Read the model definition and answer for the solid it produces. Units are mm, in the model's axes. Face numbers are marked on the shaded views. A direction names the side the tool comes from. Coordinates: 2 decimals unless noted, no trailing zeros. Write item = value, one per line.
from build123d import *

# Parameters (mm, degrees)
BOSS_EXTRUDE1_DEPTH  = 17.5
CUT_EXTRUDE1_DEPTH   = 15.5
CUT_EXTRUDE3_REACH   = 38.949
SKETCH4_R            = 8
SKETCH4_4_R          = 1
SKETCH4_4_W          = 20
SKETCH4_4_H          = 5
BOSS_EXTRUDE2_DEPTH  = 7
FILLET1_R            = 1
FILLET2_R            = 1.5
BOSS_EXTRUDE3_DEPTH  = 2
SKETCH6_W            = 11
SKETCH6_H            = 2
BOSS_EXTRUDE4_DEPTH  = 0.75
SKETCH11_R           = 8
BOSS_EXTRUDE11_DEPTH = 0.5
SKETCH14_W           = 11
SKETCH14_H           = 11
BOSS_EXTRUDE12_DEPTH = 2
BOSS_EXTRUDE13_DEPTH = 1
SKETCH6_4_W          = 11
SKETCH6_4_H          = 2.5
CUT_EXTRUDE6_DEPTH   = 0.3
SKETCH16_W           = 11
SKETCH16_H           = 2
BOSS_EXTRUDE14_DEPTH = 0.75
SKETCH16_3_W         = 11
SKETCH16_3_H         = 2.5
CUT_EXTRUDE7_DEPTH   = 0.3
CUT_EXTRUDE8_REACH   = 59.044
FILLET3_R            = 1
CHAMFER1_SIZE        = 0.5
CHAMFER3_SIZE        = 1


with BuildPart() as part:
    # Sketch1 → Boss-Extrude1 (new body)
    with BuildSketch(Plane(origin=(0, 0, 0), x_dir=(1, 0, 0), z_dir=(0, 1, 0))):
        Polygon((-15, 20), (15, 20), (15, -20), (15, -30), (-15, -30), (-15, -20), align=None)
    extrude(amount=BOSS_EXTRUDE1_DEPTH)

    # Sketch2 → Cut-Extrude1 (cut)
    with BuildSketch(Plane(origin=(0, 17.5, 0), x_dir=(1, 0, 0), z_dir=(0, 1, 0))):
        Polygon((-13, 18), (13, 18), (13, -18), (13, -28), (-13, -28), (-13, -18), align=None)
    extrude(amount=-CUT_EXTRUDE1_DEPTH, mode=Mode.SUBTRACT)

    # Sketch4 → Cut-Extrude3 (cut, up to next)
    with BuildSketch(Plane(origin=(0, 2, 0), x_dir=(1, 0, 0), z_dir=(0, 1, 0)), mode=Mode.PRIVATE) as cut_extrude3_sk1:
        with Locations(Location((0, 3.5, 0), (0, 0, 270))):
            Circle(SKETCH4_R)
    cut_extrude3_tool1 = extrude(cut_extrude3_sk1.sketch, amount=-CUT_EXTRUDE3_REACH, mode=Mode.PRIVATE) & part.part
    add(cut_extrude3_tool1.solids().sort_by_distance((0, 2, -3.5))[0], mode=Mode.SUBTRACT)

    # Sketch4<4> → Boss-Extrude2 (add)
    # profile 1 of 2: a face of its own
    with BuildSketch(Plane(origin=(0, 2, 0), x_dir=(1, 0, 0), z_dir=(0, 1, 0))):
        Polygon((10, 16), (-10, 16), (-10, 11), (-5.998750655, 11), (-3.877430311, 13.121320344), (3.877430311, 13.121320344), (5.998750655, 11), (10, 11), align=None)
        with Locations(Location((-7.5, 13.5, 0), (0, 0, 270))):
            Circle(SKETCH4_4_R, mode=Mode.SUBTRACT)
        with Locations(Location((7.5, 13.5, 0), (0, 0, 270))):
            Circle(SKETCH4_4_R, mode=Mode.SUBTRACT)
    # profile 2 of 2: a face of its own
    with BuildSketch(Plane(origin=(0, 2, 0), x_dir=(1, 0, 0), z_dir=(0, 1, 0))):
        with Locations((0, -13.5)):
            Rectangle(SKETCH4_4_W, SKETCH4_4_H)
        with Locations(Location((7.5, -13.5, 0), (0, 0, 270))):
            Circle(SKETCH4_4_R, mode=Mode.SUBTRACT)
        with Locations(Location((-7.5, -13.5, 0), (0, 0, 270))):
            Circle(SKETCH4_4_R, mode=Mode.SUBTRACT)
    extrude(amount=BOSS_EXTRUDE2_DEPTH)

    # Fillet1
    fillet1_edges = [part.edges().sort_by_distance(p)[0] for p in [
        (-4.938090483, 2, -12.060660172),
        (0, 2, -13.121320344),
        (-10, 2, -13.5),
        (-7.999375327, 2, -11),
        (0, 2, -16),
        (10, 2, -13.5),
        (7.999375327, 2, -11),
        (4.938090483, 2, -12.060660172),
        (-10, 2, 13.5),
        (0, 2, 16),
        (0, 2, 11),
        (10, 2, 13.5),
    ]]
    fillet(fillet1_edges, radius=FILLET1_R)

    # Fillet2
    fillet2_edges = [part.edges().sort_by_distance(p)[0] for p in [
        (15, 8.75, 30),
        (-15, 8.75, 30),
        (-15, 8.75, -20),
        (15, 8.75, -20),
        (0, 0, 30),
        (-15, 0, 5),
        (0, 0, -20),
        (15, 0, 5),
    ]]
    fillet(fillet2_edges, radius=FILLET2_R)

    # Sketch5 → Boss-Extrude3 (add)
    with BuildSketch(Plane(origin=(-13, 0, 0), x_dir=(0, 0, -1), z_dir=(1, 0, 0))):
        Polygon((-12, 17.5), (-18, 17.5), (-23, 17.5), (-23, 12), (-12, 12), align=None)
        Polygon((-23, 17.5), (-18, 17.5), (-12, 17.5), (-12, 23), (-23, 23), align=None)
    extrude(amount=BOSS_EXTRUDE3_DEPTH)

    # Sketch6 → Boss-Extrude4 (add)
    with BuildSketch(Plane.ZY.offset(13)):
        with Locations((17.5, 22)):
            Rectangle(SKETCH6_W, SKETCH6_H)
    extrude(amount=BOSS_EXTRUDE4_DEPTH)

    # Sketch11 → Boss-Extrude11 (add)
    with BuildSketch(Plane.XZ):
        Polygon((-12, 17), (-12, -17), (12, -17), (12, 17), (12, 27), (-12, 27), align=None)
        with Locations(Location((0, -3.5, 0), (0, 0, 90))):
            Circle(SKETCH11_R, mode=Mode.SUBTRACT)
    extrude(amount=BOSS_EXTRUDE11_DEPTH)

    # Sketch14 → Boss-Extrude12 (add)
    with BuildSketch(Plane.ZY.offset(-13)):
        with Locations((-7.5, 17.5)):
            Rectangle(SKETCH14_W, SKETCH14_H)
    extrude(amount=BOSS_EXTRUDE12_DEPTH)

    # Sketch15 → Boss-Extrude13 (add)
    with BuildSketch(Plane(origin=(0, 17.5, 0), x_dir=(1, 0, 0), z_dir=(0, 1, 0))):
        with BuildLine():
            Line((-13, -28), (-13, 18))
            Line((-13, 18), (-14, 18))
            Line((-14, 18), (-14, -29))
            Line((-14, -29), (-3, -29))
            ThreePointArc((-3, -29), (-2.998349642, -28.900504153), (-2.993400384, -28.801117774))
            Line((-2.993400384, -28.801117774), (-2.993400384, -28))
            Line((-2.993400384, -28), (-13, -28))
        make_face()
        Polygon((14, 18), (13, 18), (13, -28), (3, -28), (3, -29), (14, -29), align=None)
    extrude(amount=BOSS_EXTRUDE13_DEPTH)

    # Sketch6<4> → Cut-Extrude6 (cut)
    with BuildSketch(Plane.ZY.offset(13)):
        with Locations((17.5, 19.75)):
            Rectangle(SKETCH6_4_W, SKETCH6_4_H)
    extrude(amount=-CUT_EXTRUDE6_DEPTH, mode=Mode.SUBTRACT)

    # Sketch16 → Boss-Extrude14 (add)
    with BuildSketch(Plane(origin=(13, 0, 0), x_dir=(0, 0, -1), z_dir=(1, 0, 0))):
        with Locations((7.5, 22)):
            Rectangle(SKETCH16_W, SKETCH16_H)
    extrude(amount=BOSS_EXTRUDE14_DEPTH)

    # Sketch16<3> → Cut-Extrude7 (cut)
    with BuildSketch(Plane(origin=(13, 0, 0), x_dir=(0, 0, -1), z_dir=(1, 0, 0))):
        with Locations((7.5, 19.75)):
            Rectangle(SKETCH16_3_W, SKETCH16_3_H)
    extrude(amount=-CUT_EXTRUDE7_DEPTH, mode=Mode.SUBTRACT)

    # Sketch17 → Cut-Extrude8 (cut, up to next)
    with BuildSketch(Plane.XY.offset(30), mode=Mode.PRIVATE) as cut_extrude8_sk1:
        with BuildLine():
            Line((-3, 17.5), (3, 17.5))
            ThreePointArc((3, 17.5), (0, 14.5), (-3, 17.5))
        make_face()
    cut_extrude8_tool1 = extrude(cut_extrude8_sk1.sketch, amount=-CUT_EXTRUDE8_REACH, mode=Mode.PRIVATE) & part.part
    add(cut_extrude8_tool1.solids().sort_by_distance((0, 16.22676, 30))[0], mode=Mode.SUBTRACT)

    # Fillet3
    fillet3_edges = [part.edges().sort_by_distance(p)[0] for p in [
        (-11, 23, 17.5),
        (-13.75, 23, 17.5),
        (11, 23, -7.5),
        (13.75, 23, -7.5),
    ]]
    fillet(fillet3_edges, radius=FILLET3_R)

    # Chamfer1
    chamfer1_edges = [part.edges().sort_by_distance(p)[0] for p in [
        (0, -0.5, 27),
        (12, -0.5, 5),
        (-12, -0.5, 5),
        (0, -0.5, -17),
    ]]
    chamfer(chamfer1_edges, length=CHAMFER1_SIZE - 0.0001)  # a hair under: the kernel refuses the full size

    # Chamfer3
    chamfer3_edges = [part.edges().sort_by_distance(p)[0] for p in [
        (0, -0.5, -11.5),
    ]]
    chamfer(chamfer3_edges, length=CHAMFER3_SIZE)


solid = part.part
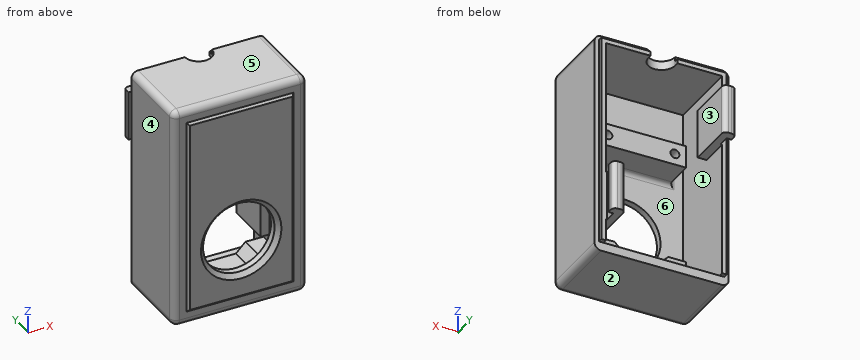
1) Flat-ended cylindrical pins translate along their axes: pin 1 Ø4 at (x, z) = (2.5, 12.5) entering from +Y; pin 2 Ø0.5 at (y, z) = (18, 0) entering from -X; pin 3 Ø11 at (y, z) = (19, 19.5) entering from +X; pin 4 Ø1 at (x, z) = (-3.5, -11) entering from -Y. Find the tip coordinate at first contact, or state that the pin passes through.
Returned:
pin_1 = 9
pin_2 = -14
pin_3 = 15
pin_4 = -0.28
2) For the marked faces 1, 2 and 3, determine the directions among +Z, -Z, +X, -X, +Y, -Y from which every point of the face is accessible in a straight line to the end or side of a thin tool.
Returned:
face_1 = none
face_2 = -Z, +X, -X, +Y, -Y
face_3 = +Y
3) Straight lines are drawn through the part: line 1 along X through (y, z) = (6.5, 13.5); line 2 along Z through (x, y) = (-12.75, 17); line 3 along Z through (x, y) = (10.75, 11.75). For each, find the intervals that lie inside material, in ascending order. Write a range as from..to.
Returned:
line_1 = -15..-13, -10..-8.5, -6.5..6.5, 8.5..10, 13..15
line_2 = -20..-18, 12..23, 28..30
line_3 = -20..-18, 28..30
4) Determine the mould class of the marked faces 4, 5 and 6 for opening direction Z: pulls with the +Z half, pulls with the -Z half, needs draft (parallel to the pull), parting line crosses it, or undercut.
Returned:
face_4 = needs draft
face_5 = pulls with the +Z half
face_6 = undercut
